Here's how the part is built. I have some questions about the finished solid (model axes, mm). A direction names the side the tool comes from. Give positions to 0.01 mm unless a question says otherwise; leave off trailing zeros. Write each loop counter-clockwise with the first axis right and the second up, starting at its lowest first coordinate (ties: lowest second). Pieces come first, ordered by that corner, then holes. Notation, with made-up numbers: (-3, 52) -> (37, 52) arc R31 cw to (37, 82) -> close; hole circle Ø4 at (-31.5, 3.25). An arc over 180 degrees is marked (long way). Use CSV: the item, a comma, the result in double quotes. Start each with the question number.
(1) If we mould it in two halves opening along Z, with no side actions, what happens to faces 1 (the flat face through (0, -6.2, 0)), 2 (the flat face through (-1.5, 8, 1)), 3 (the flat face through (0, -6.2, 1.5))? For each: pulls with the +Z half, pulls with the -Z half, needs draft (parallel to the pull), parting line crosses it, or undercut.
(2) I need wall thicknesses on L1, parallel to Y at x = 0, z = 0.4; L2, parallel to Y at x = -2.75, z = 1.4. Which ranges of each line are inside material? Lowest first, please. Write a range as [from, to].
(3) For pin 1 Ø0.8 at (y, z) = (8.5, 0.5) entering from +X; pin 2 Ø0.8 at (x, z) = (4, 0.5) entering from -Y; pin 3 Ø0.8 at (y, z) = (-7.5, 0.5) entering from -X, each with a flat end and sliding along its axis, tell me the tip position at first contact or that it passes through.
(4) Suppose I cut it at C-C on z = 0.65. List the corners of the cut face in (x, y) for me, plus the area to 3 significant figures.
(5) Suppose I cut it at A-A on x = 5.5. List the corners of the cut face in (y, z) for me.
(6) Which directions (+Z, -Z, +X, -X, +Y, -Y) give clear straight access to the entire face, cutting with the end or side of a thin tool? Please do faces 4 (the flat face through (-4, 7, 1)), 5 (the flat face through (-1.5, -8, 1)), 6 (the flat face through (0, 6, 1)).
from build123d import *

# Parameters (mm, degrees)
SKETCH_6_W          = 14
SKETCH_6_H          = 14
SKETCH_6_W_2        = 12
SKETCH_6_H_2        = 12
EXTRUDE_3_DEPTH     = 1.5
SKETCH_7_W          = 3
SKETCH_7_H          = 1.5
EXTRUDE_4_DEPTH     = 3.5
CUT_EXTRUDE_3_DEPTH = 4
SKETCH_11_R         = 1
CUT_EXTRUDE_5_DEPTH = 4


with BuildPart() as part:
    # 草图6 → 凸台-拉伸3 (new body)
    with BuildSketch(Plane.XY):
        Rectangle(SKETCH_6_W, SKETCH_6_H)
        Rectangle(SKETCH_6_W_2, SKETCH_6_H_2, mode=Mode.SUBTRACT)
    extrude(amount=EXTRUDE_3_DEPTH)

    # 草图7 → 凸台-拉伸4 (add)
    with BuildSketch(Plane.XZ.offset(7)):
        with Locations((0, 0.75)):
            Rectangle(SKETCH_7_W, SKETCH_7_H)
    extrude_4 = extrude(amount=EXTRUDE_4_DEPTH)

    # 草图8 → 切除-拉伸3 (cut)
    with BuildSketch(Plane.XY.offset(1.5)):
        with BuildLine():
            ThreePointArc((0, -10.5), (-1.060660172, -10.060660172), (-1.5, -9))
            Line((-1.5, -9), (-1.5, -10.5))
            Line((-1.5, -10.5), (0, -10.5))
        make_face()
        with BuildLine():
            Line((1.5, -10.5), (1.5, -9))
            ThreePointArc((1.5, -9), (1.060660172, -10.060660172), (0, -10.5))
            Line((0, -10.5), (1.5, -10.5))
        make_face()
    cut_extrude_3 = extrude(amount=-CUT_EXTRUDE_3_DEPTH, mode=Mode.SUBTRACT)

    # 草图11 → 切除-拉伸5 (cut)
    with BuildSketch(Plane.XY.offset(1.5)):
        with Locations((0, -9)):
            Circle(SKETCH_11_R)
    cut_extrude_5 = extrude(amount=-CUT_EXTRUDE_5_DEPTH, mode=Mode.SUBTRACT)

    # 镜向1: 凸台-拉伸4, 切除-拉伸3, 切除-拉伸5 across plane
    add(extrude_4.mirror(Plane.ZX))
    add(cut_extrude_3.mirror(Plane.ZX), mode=Mode.SUBTRACT)
    add(cut_extrude_5.mirror(Plane.ZX), mode=Mode.SUBTRACT)


solid = part.part
Geometry says:
1,face 1,"pulls with the -Z half"
1,face 2,"needs draft"
1,face 3,"pulls with the +Z half"
2,L1,"[-10.5, -10], [-8, -6], [6, 8], [10, 10.5]"
2,L2,"[-7, -6], [6, 7]"
3,pin 1,"x = 1.5"
3,pin 2,"y = -7"
3,pin 3,"x = -1.5"
4,outline,"(-7, -7) -> (-1.5, -7) -> (-1.5, -9) arc R1.5 ccw to (1.5, -9) -> (1.5, -7) -> (7, -7) -> (7, 7) -> (1.5, 7) -> (1.5, 9) arc R1.5 ccw to (-1.5, 9) -> (-1.5, 7) -> (-7, 7) -> close; hole (-6, -6) -> (6, -6) -> (6, 6) -> (-6, 6) -> close; hole circle Ø2 at (0, -9); hole circle Ø2 at (0, 9)"
4,area,"64.8 mm²"
5,outline,"(-7, 0) -> (-6, 0) -> (-6, 1.5) -> (-7, 1.5) -> close; (6, 0) -> (7, 0) -> (7, 1.5) -> (6, 1.5) -> close"
6,face 4,"+Z, -Z, -X, +Y"
6,face 5,"+Z, -Z, -X, -Y"
6,face 6,"+Z, -Z"
